```python
from build123d import *

# Parameters (mm, degrees)
F0_W     = 55.4524268955
F0_H     = 89.5769931376
F1_DEPTH = 25.4
F2_R     = 5.08
F3_R     = 18.0864233447
F4_DEPTH = 25.4
F5_T     = -2.54


with BuildPart() as f1:
    # F0 (on Top) → F1 (new body)
    with BuildSketch(Plane.XY):
        with Locations((-2.3697623983, -1.1848751456)):
            Rectangle(F0_W, F0_H)
    extrude(amount=-F1_DEPTH)

    # F2
    f2_edges = [f1.edges().sort_by_distance(p)[0] for p in [
        (-30.095976, 43.603621, -12.7),
    ]]
    fillet(f2_edges, radius=F2_R)

    # F3 (on face) → F4 (cut)
    with BuildSketch(Plane(origin=(0, 0, -25.4), x_dir=(1, 0, 0), z_dir=(0, 0, -1))):
        Circle(F3_R)
    extrude(amount=-F4_DEPTH, mode=Mode.SUBTRACT)

    # F5
    f5_openings = [f1.faces().sort_by_distance(p)[0] for p in [
        (0.170238, 42.550103, -25.4),
    ]]
    offset(amount=F5_T, openings=f5_openings)


solid = f1.part
```
The model under review builds one solid part; all positions refer to its coordinate system, in mm. A direction names the side the tool comes from. Round coordinates to 2 decimals unless told otherwise and drop trailing zeros. Loops run counter-clockwise (first coordinate to the right, second up) from the corner with the lowest first, then second, coordinate; pieces in that order, holes last. Notation, with made-up numbers: (-17, 76.5) - (19, 76.5) arc R10 cw to (19, 83.5) - close; hole circle Ø2 at (-38.5, 37.5). An arc over 180 degrees is marked (long way). Write each question's results on one line, items separated by ' | '. Start each with the question number.
Q1. Take a section at D-D on y = -25. Give the boundary of the cut face in (x, z), plus the area to 3 significant figures.
Q2. Take a section at C-C on x = 0. Give the boundary of the cut face in (y, z).
Q3. Take a section at A-A on z = -4.5. Give the boundary of the cut face in (x, y).
Q4. Draft analysis for pull direction X (two halves, no side actions). For faces 1 (the flat face through (0, 43.604, -13)), 2 (the flat face through (-30.096, -4, -13)), 3 (the flat face through (-1, 41.064, -14)), state which applies: pulls with the +X half, pulls with the -X half, needs draft (parallel to the pull), parting line crosses it, or undercut.
Q5. Take a section at B-B on y = 0. Give the boundary of the cut face in (x, z), plus the area to 3 significant figures.
Q6. Tool access review of faces 4 (the flat face through (-20, -10, -2.54)), 5 (the flat face through (-0.1, -18.24, -25.4)): name each direction out of +Z, -Z, +X, -X, +Y, -Y from which nothing blocks a thin tool from reaching the whole face with its end or side.
Q7. Insertion check: P1, Ø6, axis at x = 10, y = -35.5, coming from the -Z side. The pin has a flat end and moves straight along its axis. Give the tip position at first contact, or say it passes through.
Q8. Wall thickness on line 1 along X through (y, z) = (0, -10.25); line 2 along Y through (x, z) = (0, -19.25); line 3 along X through (y, z) = (-28, -23.75): over which ranges is each line inside the solid? List them lowest first. Write a range as [from, to].
Data:
1) outline: (-30.1, -25.4) - (-27.56, -25.4) - (-27.56, -2.54) - (22.82, -2.54) - (22.82, -25.4) - (25.36, -25.4) - (25.36, 0) - (-30.1, 0) - close | area: 257 mm²
2) outline: (-45.97, -25.4) - (-43.43, -25.4) - (-43.43, -2.54) - (-20.63, -2.54) - (-20.63, -25.4) - (-18.09, -25.4) - (-18.09, 0) - (-45.97, 0) - close; (18.09, -25.4) - (20.63, -25.4) - (20.63, -2.54) - (41.06, -2.54) - (41.06, -25.4) - (43.6, -25.4) - (43.6, 0) - (18.09, 0) - close
3) outline: (-30.1, -45.97) - (25.36, -45.97) - (25.36, 43.6) - (-25.02, 43.6) arc R5.08 ccw to (-30.1, 38.52) - close; circle Ø41.25 at (0, 0); hole (-27.56, -43.43) - (22.82, -43.43) - (22.82, 41.06) - (-25.02, 41.06) arc R2.54 ccw to (-27.56, 38.52) - close; hole circle Ø36.17 at (0, 0)
4) face 1: needs draft | face 2: pulls with the -X half | face 3: undercut
5) outline: (-30.1, -25.4) - (-27.56, -25.4) - (-27.56, -2.54) - (-20.63, -2.54) - (-20.63, -25.4) - (-18.09, -25.4) - (-18.09, 0) - (-30.1, 0) - close; (18.09, -25.4) - (20.63, -25.4) - (20.63, -2.54) - (22.82, -2.54) - (22.82, -25.4) - (25.36, -25.4) - (25.36, 0) - (18.09, 0) - close | area: 281 mm²
6) face 4: -Z | face 5: -Z, +X, -X, +Y, -Y
7) P1: stops at z = -2.54
8) line 1: x = [-30.1, -27.56], [-20.63, -18.09], [18.09, 20.63], [22.82, 25.36] | line 2: y = [-45.97, -43.43], [-20.63, -18.09], [18.09, 20.63], [41.06, 43.6] | line 3: x = [-30.1, -27.56], [22.82, 25.36]
